Autodesk Inventor part; units mm, degrees
ref_plane "nut_XY" through (0, 0, 0) normal (0, 0, -1) x (1, 0, 0)
ref_plane "nut_YZ" through (0, 0, 0) normal (1, 0, 0) x (0, -1, 0)
ref_plane "nut_ZX" through (0, 0, 0) normal (0, -1, 0) x (0, 0, -1)
sketch "Sketch_1" plane through (0, 0, 0) normal (1, 0, 0) x (0, 1, 0)
  line L0 (0, -5.588) -> (0, 0)
  line L1 (4.7625, 0) -> (3.9027, -0.8598)
  line L2 (3.9027, -0.8598) -> (3.9027, -4.7282)
  line L3 (3.9027, -4.7282) -> (4.7625, -5.588)
  line L4 (4.7625, -5.588) -> (7.112, -5.588)
  line L5 (7.112, -5.588) -> (8.5344, -5.2069)
  line L6 (8.5344, -5.2069) -> (8.5344, -0.3811)
  line L7 (8.5344, -0.3811) -> (7.112, 0)
  line L8 (7.112, 0) -> (4.7625, 0)
revolve "Revolution1" add sketch "Sketch_1" angle 360 about axis through (0, 0, -5.588) along (0, 0, -1)
thread "Thread1"
sketch "Sketch_2" plane through (0, 0, 0) normal (0, 0, 1) x (1, 0, 0)
  circle A0 centre (0, 0) radius 15.24
  line L0 (-7.112, -4.1061) -> (0, -8.2122)
  line L1 (0, -8.2122) -> (7.112, -4.1061)
  line L2 (7.112, -4.1061) -> (7.112, 4.1061)
  line L3 (7.112, 4.1061) -> (0, 8.2122)
  line L4 (0, 8.2122) -> (-7.112, 4.1061)
  line L5 (-7.112, 4.1061) -> (-7.112, -4.1061)
extrude "Extrusion1" cut sketch "Sketch_2" against normal blind 5.588
sketch "Sketch_3" plane through (7.112, 0, 0) normal (1, 0, 0) x (0, 0, -1)
  line L0 (2.159, 1.27) -> (2.159, -1.27)
  line L1 (2.159, -1.27) -> (3.429, -1.27)
  line L2 (3.429, -1.27) -> (3.429, 1.27)
  line L3 (3.429, 1.27) -> (2.159, 1.27)
extrude "Extrusion2" cut sketch "Sketch_3" along normal mid plane 0.508
sketch "Sketch_4" plane through (-3.556, 6.1592, 0) normal (0.5, -0.866, 0) x (0, 0, -1)
  line L0 (2.159, 1.27) -> (2.159, -1.27)
  line L1 (2.159, -1.27) -> (3.429, -1.27)
  line L2 (3.429, -1.27) -> (3.429, 1.27)
  line L3 (3.429, 1.27) -> (2.159, 1.27)
extrude "Extrusion3" cut sketch "Sketch_4" along normal mid plane 0.508
sketch "Sketch_5" plane through (-3.556, -6.1592, 0) normal (0.5, 0.866, 0) x (0, 0, -1)
  line L0 (2.159, 1.27) -> (2.159, -1.27)
  line L1 (2.159, -1.27) -> (3.429, -1.27)
  line L2 (3.429, -1.27) -> (3.429, 1.27)
  line L3 (3.429, 1.27) -> (2.159, 1.27)
extrude "Extrusion4" cut sketch "Sketch_5" along normal mid plane 0.508
ref_plane "nut_XY" through (0, 0, 0) normal (0, 0, -1) x (1, 0, 0)
ref_plane "nut_YZ" through (0, 0, 0) normal (1, 0, 0) x (0, -1, 0)
ref_plane "nut_ZX" through (0, 0, 0) normal (0, -1, 0) x (0, 0, -1)
properties part number "2LOPRO-NUT"
Verification items for the finished model (mm, model axes). Give positions to 0.01 mm unless a question says otherwise; leave off trailing zeros. Order: outer loops, then holes, each group sorted by start corner. A loop starts at its lowest first (then second) coordinate and runs counter-clockwise, first axis right, second up. Notation, with made-up numbers: M -19,60.5 L 34,60.5 A16 ccw 34,74.5 Z; hole C 36,48.25 d10. An arc over 180 degrees is marked long. Answer as a JSON object with one key per item and string values. Group by question number.
1) Mould release check, pull along Y, two halves, no side actions. Record for faces 1 (the face through (2.638, -2.876, -2.821)), 2 (the face through (-5, 1, -5.588)), 3 (the face through (-0.02, 7.34, -0.06)), 4 (the face through (6.4, -3.67, -0.07)): released by +Y, released by -Y, zero draft, split by the parting line, or undercut.
2) Depth check by flat-ended pin: pin 1 Ø1.6 at (x, y) = (-3.5, -6) entering from +Z; pin 2 Ø2 at (x, z) = (-4.5, -3) entering from +Y; pin 3 Ø3 at (x, z) = (1, -3) entering from -Y. Enter the tip coordinate at first touch or a pass-through.
3) Scan lines: line 1 along X through (y, z) = (0, -3.7); line 2 along X through (y, z) = (0, -2.75); line 3 along Y through (x, z) = (1.75, -3.3). Record each from-to range of solid material in increasing order. Write a range as [from, to].
4) Cross-section at A-A (z = -2.4). Enter the section's corners in (x, y), then the cut area to 3 significant figures.
5) Cross-section at B-B (z = -1.2). Enter the section's corners in (x, y), then the cut area to 3 significant figures.
Result sheet:
{
 "1": {"face 1": "undercut", "face 2": "zero draft", "face 3": "released by +Y", "face 4": "released by -Y"},
 "2": {"pin 1": "stops at z = 0", "pin 2": "stops at y = 6.14", "pin 3": "stops at y = -8.21"},
 "3": {"line 1": "x = [-7.11, -3.9], [3.9, 7.11]", "line 2": "x = [-7.11, -3.9], [3.9, 6.86]", "line 3": "y = [-7.2, -3.49], [3.49, 7.2]"},
 "4": {"outline": "M -7.11,-4.11 L -4.66,-5.52 L -4.53,-5.3 L -2.33,-6.57 L -2.46,-6.79 L 0,-8.21 L 7.11,-4.11 L 7.11,-1.27 L 6.86,-1.27 L 6.86,1.27 L 7.11,1.27 L 7.11,4.11 L 0,8.21 L -2.46,6.79 L -2.33,6.57 L -4.53,5.3 L -4.66,5.52 L -7.11,4.11 Z; hole C 0,0 d7.81", "area": "125 mm2"},
 "5": {"outline": "M -7.11,-4.11 L 0,-8.21 L 7.11,-4.11 L 7.11,4.11 L 0,8.21 L -7.11,4.11 Z; hole C 0,0 d7.81", "area": "127 mm2"}
}
